```python
from build123d import *

# Parameters (mm, degrees)
SKETCH1_R           = 1.825
BOSS_EXTRUDE1_DEPTH = 1.98
SKETCH2_R           = 0.945
BOSS_EXTRUDE2_DEPTH = 6
CUT_EXTRUDE1_DEPTH  = 1
CHAMFER1_SIZE       = 0.2


with BuildPart() as part:
    # Sketch1 → Boss-Extrude1 (new body)
    with BuildSketch(Plane(origin=(0, 0, 0), x_dir=(1, 0, 0), z_dir=(0, 1, 0))):
        Circle(SKETCH1_R)
    extrude(amount=BOSS_EXTRUDE1_DEPTH)

    # Sketch2 → Boss-Extrude2 (add)
    with BuildSketch(Plane(origin=(0, 1.98, 0), x_dir=(1, 0, 0), z_dir=(0, 1, 0))):
        Circle(SKETCH2_R)
    extrude(amount=BOSS_EXTRUDE2_DEPTH)

    # Sketch3 → Cut-Extrude1 (cut)
    with BuildSketch(Plane.XZ):
        Polygon((0.458993464, -0.795), (0.917986928, 0), (0.458993464, 0.795), (-0.458993464, 0.795), (-0.917986928, 0), (-0.458993464, -0.795), align=None)
    extrude(amount=-CUT_EXTRUDE1_DEPTH, mode=Mode.SUBTRACT)

    # Chamfer1
    chamfer1_edges = [part.edges().sort_by_distance(p)[0] for p in [
        (-0.945, 7.98, 0),
    ]]
    chamfer(chamfer1_edges, length=CHAMFER1_SIZE)


solid = part.part
```
Input: part model. Units: mm. Frame: model coordinates. A direction names the side the tool comes from. Round coordinates to 2 decimals unless told otherwise and drop trailing zeros. Loops run counter-clockwise (first coordinate to the right, second up) from the corner with the lowest first, then second, coordinate; pieces in that order, holes last. Notation, with made-up numbers: (69, -20) -> (114, -20) arc R28 ccw to (114, -2) -> close; hole circle Ø5 at (56.25, 18). An arc over 180 degrees is marked (long way). Use one line per item in the form item = value. Start each with the question number.
Item 1: Section query A-A on x = 0. Return the cut outline in (y, z) (3 decimals).
Item 2: Mould query, pull axis Z, two halves, no side actions, for faces 3 (the face through (-0.205, 4.839, 0.923)), 4 (the face through (0, 1, 0)), 5 (the face through (1, 1.98, 1)). Classes: pulls with the +Z half, pulls with the -Z half, needs draft (parallel to the pull), parting line crosses it, or undercut.
Item 3: Section query B-B on y = 6.5. Return the cut outline in (x, z) (3 decimals).
Item 4: Section query D-D on z = -1.45. Return the cut outline in (x, y).
Item 5: Material intervals for L1, parallel to Y at x = -0.95, z = 1.25; L2, parallel to Y at x = -0.3, z = 0.5; L3, parallel to Z at x = -1, y = 1.75, sorted ascending. Write a range as from..to.
Item 6: Section query C-C on z = 1.05. Return the cut outline in (x, y), then the cut area to 3 significant figures.
Item 7: Contact query for a flat-ended pin moving along its axis: pin 1 Ø1.5 at (x, y) = (-0.5, 7) entering from -Z (3 decimals). Output: stop coordinate, or through.
Item 8: Set-up query: faces 1 (the face through (0, 0.5, 0.795)), 2 (the face through (0, 0, -1)). Return all of +Z, -Z, +X, -X, +Y, -Y with unobstructed straight access to the full face (end or side cutting, diameter ignored); none if empty.
Ans:
q1.outline = (0, -1.825) -> (1.98, -1.825) -> (1.98, -0.945) -> (7.78, -0.945) -> (7.98, -0.745) -> (7.98, 0.745) -> (7.78, 0.945) -> (1.98, 0.945) -> (1.98, 1.825) -> (0, 1.825) -> (0, 0.795) -> (1, 0.795) -> (1, -0.795) -> (0, -0.795) -> close
q2.face_3 = parting line crosses it
q2.face_4 = undercut
q2.face_5 = needs draft
q3.outline = circle Ø1.89 at (0, 0)
q4.outline = (-1.11, 0) -> (1.11, 0) -> (1.11, 1.98) -> (-1.11, 1.98) -> close
q5.L1 = 0..1.98
q5.L2 = 1..7.98
q5.L3 = -1.53..1.53
q6.outline = (-1.49, 0) -> (1.49, 0) -> (1.49, 1.98) -> (-1.49, 1.98) -> close
q6.area = 5.91 mm^2
q7.pin_1 = -0.945
q8.face_1 = -Y
q8.face_2 = +Z, -Z, +X, -X, -Y
